```python
from build123d import *

# Parameters (mm, degrees)
F0_W     = 11
F0_H     = 11
F0_R     = 5
F1_DEPTH = 7
F2_DEPTH = 13
F3_R     = 4
F4_DEPTH = 4


with BuildPart() as f1:
    # F0 (on Top) → F1 (new body)
    with BuildSketch(Plane.XY):
        Rectangle(F0_W, F0_H)
        Circle(F0_R, mode=Mode.SUBTRACT)
        Circle(F0_R)
        Polygon((2, -19.5), (5.5, -5.5), (-5.5, -5.5), (-2, -19.5), align=None)
        Polygon((5.5, 5.5), (5.5, -5.5), (19.5, -2), (19.5, 2), align=None)
        Polygon((-19.5, -2), (-5.5, -5.5), (-5.5, 5.5), (-19.5, 2), align=None)
        Polygon((-5.5, 5.5), (5.5, 5.5), (2, 19.5), (-2, 19.5), align=None)
    extrude(amount=F1_DEPTH)

    # F0 (on Top) → F2 (join)
    with BuildSketch(Plane.XY):
        Circle(F0_R)
    extrude(amount=-F2_DEPTH)

    # F3 (on face) → F4 (join)
    with BuildSketch(Plane.XY.offset(7)):
        Circle(F3_R)
    extrude(amount=F4_DEPTH)


solid = f1.part
```
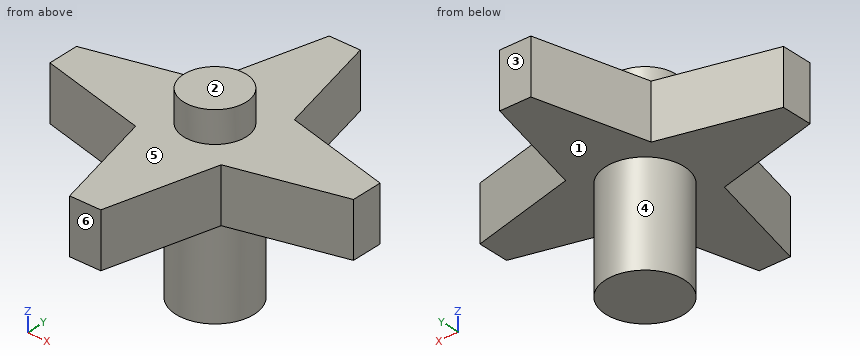
Design review of the part built by this model. Coordinates are the model's own, in mm. Face numbers are marked on the shaded views. A direction names the side the tool comes from. Coordinates: 2 decimals unless noted, no trailing zeros. Order: outer loops, then holes, each group sorted by start corner. A loop starts at its lowest first (then second) coordinate and runs counter-clockwise, first axis right, second up. Notation, with made-up numbers: (48.25, 67.25) - (78.25, 67.25) arc R34 ccw to (78.25, 103.25) - close; hole circle Ø10 at (61.25, 31.25). An arc over 180 degrees is marked (long way). One line per question, with ' | ' between items.
Q1. The part is to be moulded in two halves that separate along Z. For the marked faces 1, 2 and 3, say which applies: +Z half, -Z half, draft (parallel to the pull), parting line (faces both ways), or undercut.
Answer key:
face 1: -Z half | face 2: +Z half | face 3: draft
Q2. Consider section B-B, the plane z = 1. Give the boundary of the cut face in (x, y), then the cut area to 3 significant figures.
Answer key:
outline: (-19.5, -2) - (-5.5, -5.5) - (-2, -19.5) - (2, -19.5) - (5.5, -5.5) - (19.5, -2) - (19.5, 2) - (5.5, 5.5) - (2, 19.5) - (-2, 19.5) - (-5.5, 5.5) - (-19.5, 2) - close | area: 541 mm2
Q3. Clearance check with flat-ended pins moving along their axes: pin 1 Ø3 at (x, z) = (-8, 5) entering from -Y; pin 2 Ø10 at (x, y) = (4, 8.5) entering from +Z; pin 3 Ø3 at (y, z) = (13.5, 4.5) entering from -X (3 decimals); pin 4 Ø19.5 at (x, y) = (6.5, 2.5) entering from -Z. State where each tip first meets the part, or that it passes through.
Answer key:
pin 1: stops at y = -5.25 | pin 2: stops at z = 7 | pin 3: stops at x = -3.875 | pin 4: stops at z = -13
Q4. To check wall thickness, follow line 1 along Z through (x, y) = (-6, 4.5); line 2 along X through (y, z) = (6.5, 4); line 3 along X through (y, z) = (6, 4.5) (3 decimals). State the ranges of each line that lie inside material, in increasing order.
Answer key:
line 1: z = 0 to 7 | line 2: x = -5.25 to 5.25 | line 3: x = -5.375 to 5.375
Q5. For the marked faces 4, 5 and 6, list the 3-axis set-ups (+Z, -Z, +X, -X, +Y, -Y) from which the entire face can be reached by the end or side of a thin tool; tool diameter is ignored.
Answer key:
face 4: -Z | face 5: +Z | face 6: +Z, -Z, +X, -X, -Y
Q6. Consider section D-D, the plane z = 8.25. Give the boundary of the cut face in (x, y), then the cut area to 3 significant figures.
Answer key:
outline: circle Ø8 at (0, 0) | area: 50.3 mm2
Q7. Consider section C-C, the plane x = 17.5. Give the boundary of the cut face in (y, z), then the cut area to 3 significant figures.
Answer key:
outline: (-2.5, 0) - (2.5, 0) - (2.5, 7) - (-2.5, 7) - close | area: 35.0 mm2
Q8. Consider section A-A, the plane y = 0. Give the boundary of the cut face in (x, z), then the cut area to 3 significant figures.
Answer key:
outline: (-19.5, 0) - (-5, 0) - (-5, -13) - (5, -13) - (5, 0) - (19.5, 0) - (19.5, 7) - (4, 7) - (4, 11) - (-4, 11) - (-4, 7) - (-19.5, 7) - close | area: 435 mm2
